The listing builds one solid part. Answer for the finished solid, in the listing's coordinates (mm). Face numbers are marked on the shaded views. Give positions to 0.01 mm unless a question says otherwise; leave off trailing zeros. Order: outer loops, then holes, each group sorted by start corner. A loop starts at its lowest first (then second) coordinate and runs counter-clockwise, first axis right, second up. Notation, with made-up numbers: (-38.5, -23.75) -> (-9.5, -23.75) arc R6 ccw to (-9.5, -17.75) -> close; hole circle Ø2 at (34, -22). An arc over 180 degrees is marked (long way). Answer as a JSON object with one key per item and string values. Group by question number.
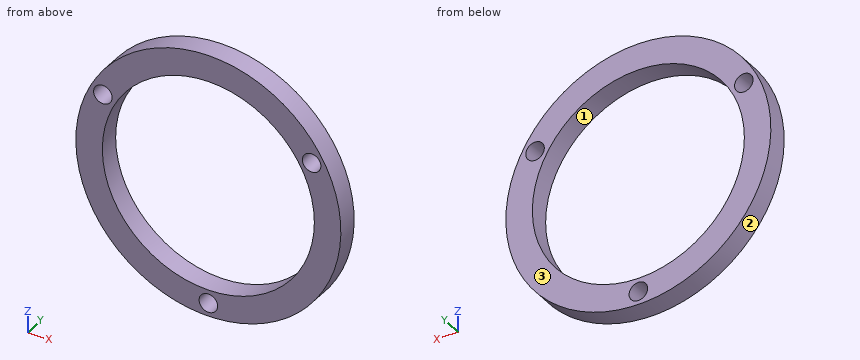
```python
from build123d import *

# Parameters (mm, degrees)
SKIZZE2_R                       = 50
SKIZZE2_R_2                     = 2
AUFSATZ_LINEAR_AUSTRAGEN1_DEPTH = 8
SCHNITT_LINEAR_AUSTRAGEN2_DEPTH = 3
SKIZZE39_R                      = 40
SCHNITT_LINEAR_AUSTRAGEN3_DEPTH = 10
SKIZZE10_R                      = 3.5
SCHNITT_LINEAR_AUSTRAGEN4_DEPTH = 10


with BuildPart() as part:
    # Skizze2 → Aufsatz-Linear austragen1 (new body)
    with BuildSketch(Plane(origin=(0, 0, 0), x_dir=(1, 0, 0), z_dir=(0, 1, 0))):
        with Locations(Location((0, 0, 0), (0, 0, 270))):
            Circle(SKIZZE2_R)
        with Locations(Location((38.97114317, -22.5, 0), (0, 0, 270))):
            Circle(SKIZZE2_R_2, mode=Mode.SUBTRACT)
        with Locations(Location((-39.80150929, -20.996186754, 0), (0, 0, 270))):
            Circle(SKIZZE2_R_2, mode=Mode.SUBTRACT)
        with Locations(Location((0, 45, 0), (0, 0, 270))):
            Circle(SKIZZE2_R_2, mode=Mode.SUBTRACT)
        with Locations(Location((0, -35, 0), (0, 0, 270))):
            Circle(SKIZZE2_R_2, mode=Mode.SUBTRACT)
        with Locations(Location((0, -27.5, 0), (0, 0, 270))):
            Circle(SKIZZE2_R_2, mode=Mode.SUBTRACT)
    extrude(amount=AUFSATZ_LINEAR_AUSTRAGEN1_DEPTH)

    # Skizze9 → Schnitt-Linear austragen2 (cut)
    with BuildSketch(Plane(origin=(0, 8, 0), x_dir=(1, 0, 0), z_dir=(0, 1, 0))):
        with BuildLine():
            Line((-6, -39.531216002), (-6, -22.531216002))
            Line((-6, -22.531216002), (6, -22.531216002))
            Line((6, -22.531216002), (6, -39.531216002))
            ThreePointArc((6, -39.531216002), (0, 39.983959767), (-6, -39.531216002))
        make_face()
    extrude(amount=-SCHNITT_LINEAR_AUSTRAGEN2_DEPTH, mode=Mode.SUBTRACT)

    # Skizze39 → Schnitt-Linear austragen3 (cut)
    with BuildSketch(Plane(origin=(0, 0, 0), x_dir=(-1, 0, 0), z_dir=(0, -1, 0))):
        with Locations(Location((0, 0, 0), (0, 0, 90))):
            Circle(SKIZZE39_R)
    extrude(amount=-SCHNITT_LINEAR_AUSTRAGEN3_DEPTH, mode=Mode.SUBTRACT)

    # Skizze10 → Schnitt-Linear austragen4 (cut)
    with BuildSketch(Plane.XZ):
        with Locations(Location((38.97114317, 22.5, 0), (0, 0, 270))):
            Circle(SKIZZE10_R)
        with Locations(Location((-39.80150929, 20.996186754, 0), (0, 0, 270))):
            Circle(SKIZZE10_R)
        with Locations(Location((0, -45, 0), (0, 0, 270))):
            Circle(SKIZZE10_R)
    extrude(amount=-SCHNITT_LINEAR_AUSTRAGEN4_DEPTH, mode=Mode.SUBTRACT)


solid = part.part
```
(1) Flat-ended cylindrical pins translate along their axes: pin 1 Ø1.5 at (y, z) = (3, -10.5) entering from -X; pin 2 Ø4 at (y, z) = (2, 6.5) entering from -X; pin 3 Ø1.5 at (x, y) = (-19, 5) entering from +Z. Find the tip coordinate at first contact, or state that the pin passes through.
(2) Find the intervals of material crossed by line 1 along X through (y, z) = (3.5, 0); line 2 along X through (y, z) = (3, -4.5); line 3 along X through (y, z) = (2.5, 22.5), in increasing order. Write a range as [from, to].
(3) A cutting plane is placed at A-A (x = 0). Determine the outline of the cut face in (y, z).
(4) A cutting plane is placed at B-B (z = 0). Determine the outline of the cut face in (x, y), and give its area (3 significant figures).
(5) A cutting plane is placed at D-D (y = 5). Determine the outline of the cut face in (x, z), and give its area (3 significant figures).
(6) For a pull along X with two mould halves and no side action, classify the marked faces 1, 2 and 3 as +X half, -X half, draft (parallel to the pull), parting line (faces both ways), or undercut.
(7) A cutting plane is placed at C-C (x = 22). Determine the outline of the cut face in (y, z), and give its area (3 significant figures).
Check sheet entries:
{
 "1": {"pin 1": "stops at x = -49.04", "pin 2": "stops at x = -49.8", "pin 3": "stops at z = 46.55"},
 "2": {"line 1": "x = [-50, -40], [40, 50]", "line 2": "x = [-49.8, -39.75], [39.75, 49.8]", "line 3": "x = [-44.65, -42.96], [-36.64, -33.07], [33.07, 35.47], [42.47, 44.65]"},
 "3": {"outline": "(0, -50) -> (8, -50) -> (8, -48.5) -> (0, -48.5) -> close; (0, -41.5) -> (8, -41.5) -> (8, -40) -> (0, -40) -> close; (0, 40) -> (8, 40) -> (8, 50) -> (0, 50) -> close"},
 "4": {"outline": "(-50, 0) -> (-40, 0) -> (-40, 8) -> (-50, 8) -> close; (40, 0) -> (50, 0) -> (50, 8) -> (40, 8) -> close", "area": "160 mm2"},
 "5": {"outline": "circle Ø100 at (0, 0); hole circle Ø7 at (-39.8, 21); hole circle Ø80 at (0, 0); hole circle Ø7 at (0, -45); hole circle Ø7 at (38.97, 22.5)", "area": "2,710 mm2"},
 "6": {"face 1": "undercut", "face 2": "parting line", "face 3": "draft"},
 "7": {"outline": "(0, -44.9) -> (8, -44.9) -> (8, -33.41) -> (0, -33.41) -> close; (0, 33.41) -> (8, 33.41) -> (8, 44.9) -> (0, 44.9) -> close", "area": "184 mm2"}
}
